Autodesk Fusion 360 part; units mm, degrees
sketch "Sketch1" plane through (0, 0, 0) normal (0, 0, 1) x (1, 0, 0)
  line L0 (0, 0) -> (50, 0)
  line L1 (0, 0) -> (-25, 0)
  line L2 (-47, -30) -> (50, -30)
  line L3 (-47, -30) -> (-47, -15)
  line L4 (-47, -30) -> (-47, -45)
  line L5 (-47, -15) -> (-25, 0)
  line L6 (-25, 0) -> (-25, -30)
  line L7 (-25, -30) -> (-25, -60)
  line L8 (-25, -60) -> (-47, -45)
  line L9 (-25, -60) -> (18, -60)
  line L10 (18, -60) -> (18, -30)
  line L11 (50, -30) -> (50, -60)
  circle A0 centre (50, -60) radius 12.5
  circle A1 centre (50, -60) radius 20
  line L12 (18, -60) -> (18, -80)
  line L13 (18, -80) -> (50, -80)
  line L14 (50, 0) -> (68.8562, -53.3333)
  dimension "d3" = 50
  dimension "d4" = 25
  dimension "d8" = 15
  dimension "d9" = 15
  dimension "d11" = 30
  dimension "d12" = 25
  dimension "d13" = 40
extrude "Extrude1" add sketch "Sketch1" along normal blind 55 contours L0 L1 L2 L6 L11 A1 L14 | L2 L3 L5 L6 | A0 | A1 | L2 L4 L7 L8 | L2 L7 L9 L10 | L2 L10 L11 A1 L12 L13
sketch "Sketch2" plane through (0, -80, 0) normal (0, -1, 0) x (1, 0, 0)
  line L0 (18, 0) -> (50, 0)
  line L1 (50, 0) -> (50, 55)
  line L2 (50, 55) -> (18, 55)
  line L3 (18, 55) -> (18, 0)
  line L4 (15, -0.0176) -> (15, 34.9824)
  line L5 (15, 34.9824) -> (18, 34.9824)
  circle A0 centre (18, 34.9824) radius 3
  line L6 (18, 34.9824) -> (18, 37.9824)
  line L7 (70.6384, 36.4824) -> (70.6384, -2.3651)
  line L8 (70.6384, -2.3651) -> (18, 0)
  line L9 (18, 37.9824) -> (30, 37.9824)
  line L10 (30, 37.9824) -> (71, 37.9824)
  line L11 (71, 37.9824) -> (70.6384, 36.4824)
  dimension "d17" = 35
  dimension "d19" = 3
  dimension "d20" = 6
extrude "Extrude2" cut sketch "Sketch2" against normal blind 115 contours L0 L1 L3 A0 L9 L10 | L0 L1 L7 L8 L10 L11 | L3 L5 A0 | L3 A0 L6 | L3 L5 A0 L6
sketch "Sketch3" plane through (0, -60, 0) normal (0, -1, 0) x (1, 0, 0)
  arc A0 (18, 37.9824) -> (18, 31.9824) centre (18, 34.9824) ccw
  line L0 (18, 37.9824) -> (18, 55)
  line L1 (18, 55) -> (-25, 55)
  line L2 (-25, 55) -> (-25, 0)
  line L3 (-25, 0) -> (18, 0)
  line L4 (18, 0) -> (18, 31.9824)
  line L5 (15, 34.9824) -> (18, 34.9824)
  line L6 (18, 34.9824) -> (18, 0)
  line L7 (18, 0) -> (15, 0)
  line L8 (15, 0) -> (15, 34.9824)
extrude "Extrude3" cut sketch "Sketch3" against normal blind 120 contours A0 L3 L4 L6 L7 L8
sketch "Sketch4" plane through (0, 0, 55) normal (0, 0, 1) x (-1, 0, 0)
  line L0 (-50, 0) -> (25, 0)
  line L1 (25, 0) -> (47, 15)
  line L2 (47, 15) -> (47, 45)
  line L3 (47, 45) -> (25, 60)
  line L4 (25, 60) -> (-18, 60)
  line L5 (-18, 60) -> (-18, 80)
  line L6 (-18, 80) -> (-50, 80)
  arc A0 (-50, 80) -> (-68.8562, 53.3333) centre (-50, 60) ccw
  line L7 (-68.8562, 53.3333) -> (-50, 0)
  line L8 (-50, 80) -> (-50, 60)
  line L9 (-50, 60) -> (-70, 60)
  circle A1 centre (-50, 60) radius 12.5
  dimension "d25" = 25
extrude "Extrude4" cut sketch "Sketch4" against normal blind 50 contours L8 L9 A1 | L8 L9 A1
sketch "Sketch5" plane through (0, 0, 55) normal (0, 0, 1) x (-1, 0, 0)
  circle A0 centre (-50, 60) radius 12.5
  line L0 (-50, 0) -> (25, 0)
  line L1 (25, 0) -> (47, 15)
  line L2 (47, 15) -> (47, 45)
  line L3 (47, 45) -> (25, 60)
  line L4 (25, 60) -> (-18, 60)
  line L5 (-18, 60) -> (-18, 80)
  line L6 (-18, 80) -> (-50, 80)
  arc A1 (-50, 80) -> (-68.8562, 53.3333) centre (-50, 60) ccw
  line L7 (-68.8562, 53.3333) -> (-50, 0)
  line L8 (47, 30) -> (47, 20)
  line L9 (47, 30) -> (47, 40)
  line L10 (47, 30) -> (30, 30)
  circle A2 centre (30, 30) radius 6
  line L11 (30, 30) -> (30, 24)
  line L12 (30, 30) -> (30, 36)
  line L13 (30, 30) -> (5, 30)
  circle A3 centre (5, 30) radius 6
  line L14 (30, 24) -> (5, 24)
  line L15 (30, 36) -> (5, 36)
  dimension "d28" = 10
  dimension "d29" = 10
  dimension "d30" = 17
  dimension "d31" = 12
  dimension "d32" = 25
  dimension "d33" = 12
extrude "Extrude5" cut sketch "Sketch5" against normal blind 20 contours L10 A2 L11 | L10 A2 L12 | A2 L12 L13 | A2 L11 L13 | A2 L13 A3 L15 | A2 L13 A3 L14 | A3
sketch "Sketch6" plane through (0, 0, 55) normal (0, 0, 1) x (-1, 0, 0)
  line L0 (5, 36) -> (30, 36)
  arc A0 (30, 24) -> (30, 36) centre (30, 30) ccw
  line L1 (30, 24) -> (5, 24)
  arc A1 (5, 36) -> (5, 24) centre (5, 30) ccw
  circle A2 centre (-50, 60) radius 12.5
  line L2 (-50, 0) -> (25, 0)
  line L3 (25, 0) -> (47, 15)
  line L4 (47, 15) -> (47, 45)
  line L5 (47, 45) -> (25, 60)
  line L6 (25, 60) -> (-18, 60)
  line L7 (-18, 60) -> (-18, 80)
  line L8 (-18, 80) -> (-50, 80)
  arc A3 (-50, 80) -> (-68.8562, 53.3333) centre (-50, 60) ccw
  line L9 (-68.8562, 53.3333) -> (-50, 0)
  circle A4 centre (-50, 60) radius 20
  circle A5 centre (-50, 60) radius 12.5
  dimension "d36" = 40
  dimension "d37" = 25
extrude "Extrude6" add sketch "Sketch6" along normal blind 20 contours A3 A4
sketch "Sketch7" plane through (0, -60, 0) normal (0, -1, 0) x (1, 0, 0)
  line L0 (15, 0) -> (15, 34.9824)
  arc A0 (18, 37.9824) -> (15, 34.9824) centre (18, 34.9824) ccw
  line L1 (18, 37.9824) -> (18, 55)
  line L2 (18, 55) -> (-25, 55)
  line L3 (-25, 55) -> (-25, 0)
  line L4 (-25, 0) -> (15, 0)
  line L5 (-47, 0) -> (-9, 0)
  line L6 (-9, 0) -> (-9, 20)
  circle A1 centre (-9, 20) radius 10
  dimension "d40" = 38
  dimension "d41" = 20
  dimension "d42" = 20
extrude "Extrude7" cut sketch "Sketch7" against normal blind 130 contours A1
sketch "Sketch8" plane through (0, 0, 0) normal (0, 0, -1) x (1, 0, 0)
  line L0 (15, 0) -> (15, 60)
  line L1 (15, 60) -> (-25, 60)
  line L2 (-25, 60) -> (-47, 45)
  line L3 (-47, 45) -> (-47, 15)
  line L4 (-47, 15) -> (-25, 0)
  line L5 (-25, 0) -> (15, 0)
  line L6 (-47, 30) -> (15, 30)
  line L7 (-47, 30) -> (-32, 30)
  line L8 (15, 30) -> (0, 30)
  circle A0 centre (-32, 30) radius 10
  circle A1 centre (0, 30) radius 10
  dimension "d45" = 15
  dimension "d46" = 15
  dimension "d47" = 20
  dimension "d48" = 20
extrude "Extrude8" cut sketch "Sketch8" against normal blind 35 contours L6 L8 A1 | L6 L8 A1 | L6 L7 A0 | L6 L7 A0
equation "d34 = -55.00 mm + 35 mm"
equation "d38 = 75.00 mm - 55 mm"
Part model, mm, in its own coordinate system. A direction names the side the tool comes from. Round coordinates to 2 decimals unless told otherwise and drop trailing zeros. Write each loop counter-clockwise with the first axis right and the second up, starting at its lowest first coordinate (ties: lowest second). Pieces come first, ordered by that corner, then holes. Notation, with made-up numbers: (47, -19.5) -> (89, -19.5) arc R32 cw to (89, 18.5) -> close; hole circle Ø8 at (3.5, 45.25). An arc over 180 degrees is marked (long way). Return JSON: item names as keys, results as strings. Group by question number.
Q1. Probe L1, parallel to X at y = -30, z = 28; L2, parallel to X at y = -30, z = 9.5; L3, parallel to Y at x = 0, z = 9. List the from-to ranges inside material, lowest first. Write a range as [from, to].
Q2. Which spindle directions (+Z, -Z, +X, -X, +Y, -Y) get a long thin tool onto all of the face, cutting with end or side? Do faces 1 (the flat face through (18, -70, 46)), 2 (the flat face through (38, -41, 37.982)), 3 (the flat face through (-37, -30, 35)), 4 (the cylindrical face through (33.324, -48.958, 64.86)). Say none if no direction does.
Q3. Mould opens along Y. For faces 5 (the flat face through (41, -69, 75)), 6 (the cylindrical face through (66.5, -71.3, 64.9)), 7 (the flat face through (3, -30, 35)) say: pulls with the +Y half, pulls with the -Y half, needs draft (parallel to the pull), parting line crosses it, or undercut.
Q4. Saw through at B-B on z = 14. Write the cut outline in (x, y).
Q5. Saw through at A-A on z = 43. Write the cut outline in (x, y), plus the area to 3 significant figures.
Q6. Saw through at C-C on y = -70.5. Write the cut outline in (x, z), plus the area to 3 significant figures.
Q7. Saw through at D-D on x = -1.5. Write the cut outline in (y, z), plus the area to 3 significant figures.
Q8. Pin check, flat tips, straight feed: pin 1 (5 mm diameter, centred on x = -2, y = -58.5, fed in from +Z); pin 2 (5 mm diameter, centred on x = 57.5, y = -30.5, fed in from -Z); pin 3 (5 mm diameter, centred on x = 6, z = 39, fed in from -Y). Stop position of each tip, or through.
Answer:
{
 "1": {"L1": "[-47, -42], [-22, -15], [10, 15]", "L2": "[-47, -42], [-22, -10], [10, 15]", "L3": "[-60, -40], [-20, 0]"},
 "2": {"face 1": "+Z, -Z, -X, -Y", "face 2": "-Z, +X, +Y, -Y", "face 3": "-Z", "face 4": "+Z"},
 "3": {"face 5": "needs draft", "face 6": "parting line crosses it", "face 7": "undercut"},
 "4": {"outline": "(-47, -45) -> (-25, -60) -> (-17, -60) -> (-17, 0) -> (-25, 0) -> (-47, -15) -> close; (-1, -60) -> (15, -60) -> (15, 0) -> (-1, 0) -> (-1, -20.05) arc R10 cw (long way) to (-1, -39.95) -> close; hole circle Ø20 at (-32, -30)"},
 "5": {"outline": "(-47, -45) -> (-25, -60) -> (18, -60) -> (18, -80) -> (50, -80) arc R20 ccw to (68.86, -53.33) -> (50, 0) -> (-25, 0) -> (-47, -15) -> close; hole (-30, -36) -> (-5, -36) arc R6 ccw to (-5, -24) -> (-30, -24) arc R6 ccw to start; hole circle Ø25 at (50, -60)", "area": "6,170 mm2"},
 "6": {"outline": "(18, 37.98) -> (43.22, 37.98) -> (43.22, 75) -> (32.98, 75) -> (32.98, 55) -> (18, 55) -> close; (56.78, 37.98) -> (67.02, 37.98) -> (67.02, 75) -> (56.78, 75) -> close", "area": "1,010 mm2"},
 "7": {"outline": "(-60, 0) -> (-39.89, 0) -> (-39.89, 13.39) -> (-60, 13.39) -> close; (-60, 26.61) -> (-39.89, 26.61) -> (-39.89, 35) -> (-34.87, 35) -> (-34.87, 55) -> (-60, 55) -> close; (-25.13, 35) -> (-20.11, 35) -> (-20.11, 26.61) -> (0, 26.61) -> (0, 55) -> (-25.13, 55) -> close; (-20.11, 0) -> (0, 0) -> (0, 13.39) -> (-20.11, 13.39) -> close", "area": "1,880 mm2"},
 "8": {"pin 1": "z = 55", "pin 2": "z = 37.98", "pin 3": "y = -60"}
}
